Work out the finished part from the listing and answer in its coordinate system (mm). Give positions to 0.01 mm unless a question says otherwise; leave off trailing zeros. Write each loop counter-clockwise with the first axis right and the second up, starting at its lowest first coordinate (ties: lowest second). Pieces come first, ordered by that corner, then holes. Notation, with made-up numbers: (-12, 17.25) -> (-3, 17.25) arc R13 cw to (-3, 40.25) -> close; hole circle Ø10 at (-18, -39). An arc over 180 degrees is marked (long way). Use a Markdown table: item, result. Add a question column.
Q1. Section A-A, the plane x = 57 is taken. Give the vertices of the cut face in (y, z) (3 decimals), plus the area to 3 significant figures.
Q2. Consider line 1 (X direction, y = 0.3, z = -5); line 2 (Z direction, x = 57, y = 0.65). Determine where each line is inside the solid, lowest interval first.
Q3. Section B-B, the plane z = -5 is taken. Give the vertices of the cut face in (x, y) (3 decimals).
Q4. This flat-tipped pin is pushed along its axis until it touches: pin 1 Ø3.5 at (x, z) = (57, -5) entering from +Y (3 decimals). Where does it stop, or does it pass through?
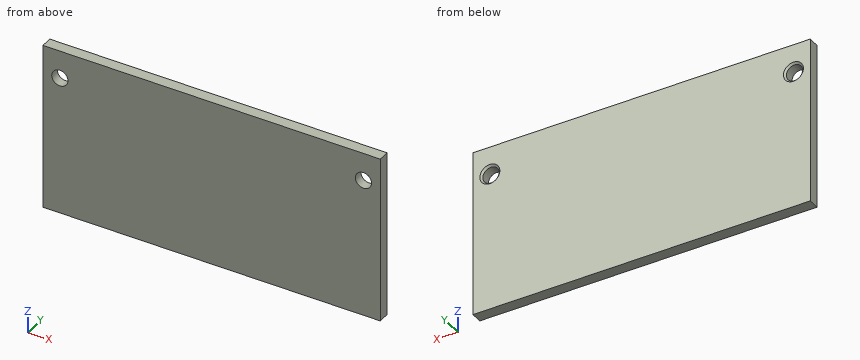
from build123d import *

# Parameters (mm, degrees)
SKETCH_1_W                     = 60
SKETCH_1_H                     = 30
EXTRUDE_1_DEPTH                = 2
HOLE_WIZARD_M3_5_1_D           = 2.9
HOLE_WIZARD_M3_5_1_CSINK_D     = 3.55
HOLE_WIZARD_M3_5_1_CSINK_ANGLE = 90


with BuildPart() as part:
    # 草图1 → 凸台-拉伸1 (new body)
    with BuildSketch(Plane(origin=(0, 0, 0), x_dir=(1, 0, 0), z_dir=(0, 1, 0))):
        with Locations((30, 15)):
            Rectangle(SKETCH_1_W, SKETCH_1_H)
    extrude(amount=EXTRUDE_1_DEPTH)

    # M3.5 螺纹孔1 (through all)
    with Locations(Plane(origin=(0, 2, 0), x_dir=(1, 0, 0), z_dir=(0, 1, 0))):
        with Locations((3, 5), (57, 5)):
            CounterSinkHole(HOLE_WIZARD_M3_5_1_D / 2, HOLE_WIZARD_M3_5_1_CSINK_D / 2, counter_sink_angle=HOLE_WIZARD_M3_5_1_CSINK_ANGLE)


solid = part.part
Result set:
| question | item | result |
|---|---|---|
| 1 | outline | (0, -30) -> (2, -30) -> (2, -6.775) -> (1.675, -6.45) -> (0, -6.45) -> close; (0, -3.55) -> (1.675, -3.55) -> (2, -3.225) -> (2, 0) -> (0, 0) -> close |
| 1 | area | 54.1 mm2 |
| 2 | line 1 | x = 0 to 1.55, 4.45 to 55.55, 58.45 to 60 |
| 2 | line 2 | z = -30 to -6.45, -3.55 to 0 |
| 3 | outline | (0, 0) -> (1.55, 0) -> (1.55, 1.675) -> (1.225, 2) -> (0, 2) -> close; (4.45, 0) -> (55.55, 0) -> (55.55, 1.675) -> (55.225, 2) -> (4.775, 2) -> (4.45, 1.675) -> close; (58.45, 0) -> (60, 0) -> (60, 2) -> (58.775, 2) -> (58.45, 1.675) -> close |
| 4 | pin 1 | stops at y = 1.975 |
